```python
from build123d import *

# Parameters (mm, degrees)
F0_R     = 4.5
F1_DEPTH = 15


with BuildPart() as f1:
    # F0 (on Front) → F1 (new body)
    with BuildSketch(Plane.XZ):
        with BuildLine():
            Line((-166.539142, 170), (-235, 170))
            Line((-235, 170), (-235, 3.228757))
            ThreePointArc((-235, 3.228757), (-226.686517, 8.849151), (-216.689655, 9.724138))
            Line((-216.689655, 9.724138), (-157.517241, -0.206897))
            ThreePointArc((-157.517241, -0.206897), (-145.051814, -16.245682), (-160, -30))
            Line((-160, -30), (-220, -30))
            ThreePointArc((-220, -30), (-228.228757, -28.228757), (-235, -23.228757))
            Line((-235, -23.228757), (-235, -170))
            Line((-235, -170), (0, -170))
            Line((0, -170), (235, -170))
            Line((235, -170), (235, -23.228757))
            ThreePointArc((235, -23.228757), (228.228757, -28.228757), (220, -30))
            Line((220, -30), (160, -30))
            ThreePointArc((160, -30), (145.051814, -16.245682), (157.517241, -0.206897))
            Line((157.517241, -0.206897), (216.689655, 9.724138))
            ThreePointArc((216.689655, 9.724138), (226.686517, 8.849151), (235, 3.228757))
            Line((235, 3.228757), (235, 170))
            Line((235, 170), (166.539142, 170))
            ThreePointArc((166.539142, 170), (152.745356, 165.850215), (143.530869, 154.778516))
            Line((143.530869, 154.778516), (76.644435, -2.601329))
            ThreePointArc((76.644435, -2.601329), (60.05836, -22.530386), (35.229544, -30))
            Line((35.229544, -30), (0, -30))
            Line((0, -30), (-35.229544, -30))
            ThreePointArc((-35.229544, -30), (-60.05836, -22.530386), (-76.644435, -2.601329))
            Line((-76.644435, -2.601329), (-143.530869, 154.778516))
            ThreePointArc((-143.530869, 154.778516), (-152.745356, 165.850215), (-166.539142, 170))
        make_face()
        with Locations((-205, 80)):
            Circle(F0_R, mode=Mode.SUBTRACT)
        with Locations((205, 80)):
            Circle(F0_R, mode=Mode.SUBTRACT)
    extrude(amount=F1_DEPTH)


solid = f1.part
```
Could you check a few things on this model? Use its own coordinates, in mm. A direction names the side the tool comes from. Round coordinates to 2 decimals unless told otherwise and drop trailing zeros. Loops run counter-clockwise (first coordinate to the right, second up) from the corner with the lowest first, then second, coordinate; pieces in that order, holes last. Notation, with made-up numbers: (-35.5, 27) - (9.5, 27) arc R24 ccw to (9.5, 58) - close; hole circle Ø4 at (33, -36). An arc over 180 degrees is marked (long way). Answer in a Markdown table with one row per item. Add a question column.
(1) If we section it at A-A (z = 48): Please give me the cut outline in (x, y), plus the area to 3 significant figures.
(2) I'm going to push flat-ended pins straight in: pin 1 (1.5 mm diameter, centred on x = 75.5, y = -10, fed in from +Z); pin 2 (1.5 mm diameter, centred on x = 72, y = -2, fed in from +Z). Where does each tip first touch, or does it pass through?
(3) If we section it at B-B (y = -9.5): Please give me the cut outline in (x, z), plus the area to 3 significant figures.
(4) If we mould it in two halves opening along Z, with no side actions, what happens to faces 4 (the face through (110.556, -7.395, 77.19)), 5 (the face through (-3, -7, -170)), 6 (the face through (-190, -7, -30)), 7 (the face through (-3, -15, -35))? For each: pulls with the +Z half, pulls with the -Z half, needs draft (parallel to the pull), parting line crosses it, or undercut.
(5) If we section it at D-D (x = 0.5): Please give me the cut outline in (y, z), plus the area to 3 significant figures.
(6) For faces 1 (the face through (-3, 0, -35)), 2 (the face through (145.08, -7.4, -16.56)), 3 (the face through (60.4, -7.4, -22.3)), which set-ups out of +Z, -Z, +X, -X, +Y, -Y let a thin tool reach every point of the face, with its end or its side?
(7) I need wall thicknesses on line 1 along Z through (x, y) = (178, -11.5); line 2 along Z through (x, y) = (205, -7); line 3 along Z through (x, y) = (-149, -2.5). Which ranges of each line are inside material? Lowest first, please.
(8) If we section it at C-C (x = 182.5): Please give me the cut outline in (y, z).
Model answer:
| question | item | result |
|---|---|---|
| 1 | outline | (-235, -15) - (-98.15, -15) - (-98.15, 0) - (-235, 0) - close; (98.15, -15) - (235, -15) - (235, 0) - (98.15, 0) - close |
| 1 | area | 4,110 mm² |
| 2 | pin 1 | stops at z = -3.5 |
| 2 | pin 2 | stops at z = -9.84 |
| 3 | outline | (-235, -170) - (235, -170) - (235, -23.23) arc R20 cw to (220, -30) - (160, -30) arc R15 cw to (157.52, -0.21) - (216.69, 9.72) arc R20 cw to (235, 3.23) - (235, 170) - (166.54, 170) arc R25 ccw to (143.53, 154.78) - (76.64, -2.6) arc R45 cw to (35.23, -30) - (-35.23, -30) arc R45 cw to (-76.64, -2.6) - (-143.53, 154.78) arc R25 ccw to (-166.54, 170) - (-235, 170) - (-235, 3.23) arc R20 cw to (-216.69, 9.72) - (-157.52, -0.21) arc R15 cw to (-160, -30) - (-220, -30) arc R20 cw to (-235, -23.23) - close; hole circle Ø9 at (-205, 80); hole circle Ø9 at (205, 80) |
| 3 | area | 111,000 mm² |
| 4 | face 4 | pulls with the +Z half |
| 4 | face 5 | pulls with the -Z half |
| 4 | face 6 | undercut |
| 4 | face 7 | needs draft |
| 5 | outline | (-15, -170) - (0, -170) - (0, -30) - (-15, -30) - close |
| 5 | area | 2,100 mm² |
| 6 | face 1 | +Z, -Z, +X, -X, +Y |
| 6 | face 2 | +Y, -Y |
| 6 | face 3 | +Z, +Y, -Y |
| 7 | line 1 | z = -170 to -30, 3.23 to 170 |
| 7 | line 2 | z = -170 to -30, 7.76 to 75.5, 84.5 to 170 |
| 7 | line 3 | z = -170 to -25.2, -4.8 to 162.82 |
| 8 | outline | (-15, -170) - (0, -170) - (0, -30) - (-15, -30) - close; (-15, 3.99) - (0, 3.99) - (0, 170) - (-15, 170) - close |
